```python
from build123d import *

# Parameters (mm, degrees)
SKETCH_1_R          = 22.25
SKETCH_1_R_2        = 2.5
EXTRUDE_1_DEPTH     = 2
SKETCH_3_R          = 11
SKETCH_3_R_2        = 2.5
EXTRUDE_3_DEPTH     = 13
EXTRUDE_START       = 6
SKETCH_4_R          = 11
EXTRUDE_4_DEPTH     = 6
SKETCH_6_R          = 2.5
CUT_EXTRUDE_2_DEPTH = 9


with BuildPart() as part:
    # 草图1 → 凸台-拉伸1 (new body)
    with BuildSketch(Plane(origin=(0, 0, 0), x_dir=(1, 0, 0), z_dir=(0, 1, 0))):
        with Locations(Location((0, 0, 0), (0, 0, 270))):
            Circle(SKETCH_1_R)
        with Locations(Location((0, 17.5, 0), (0, 0, 270))):
            Circle(SKETCH_1_R_2, mode=Mode.SUBTRACT)
        with Locations(Location((-15.155444566, -8.75, 0), (0, 0, 270))):
            Circle(SKETCH_1_R_2, mode=Mode.SUBTRACT)
        with Locations(Location((15.155444566, -8.75, 0), (0, 0, 270))):
            Circle(SKETCH_1_R_2, mode=Mode.SUBTRACT)
    extrude(amount=EXTRUDE_1_DEPTH)

    # 草图3 → 凸台-拉伸3 (add)
    with BuildSketch(Plane(origin=(0, 2, 0), x_dir=(1, 0, 0), z_dir=(0, 1, 0))):
        with Locations(Location((0, 0, 0), (0, 0, 90))):
            Circle(SKETCH_3_R)
        with Locations(Location((0, 0, 0), (0, 0, 90))):
            Circle(SKETCH_3_R_2, mode=Mode.SUBTRACT)
    extrude(amount=EXTRUDE_3_DEPTH)

    # 草图4 → 凸台-拉伸4 (add)
    with BuildSketch(Plane.XZ.offset(EXTRUDE_START)):
        with Locations(Location((0, 0, 0), (0, 0, 270))):
            Circle(SKETCH_4_R)
    extrude(amount=-EXTRUDE_4_DEPTH)

    # 草图6 → 切除-拉伸2 (cut)
    with BuildSketch(Plane.XZ.offset(6)):
        with Locations(Location((0, 0, 0), (0, 0, 270))):
            Circle(SKETCH_6_R)
    extrude(amount=-CUT_EXTRUDE_2_DEPTH, mode=Mode.SUBTRACT)


solid = part.part
```
Geometry: final body of the model. Coordinates: model frame, mm. A direction names the side the tool comes from. Give positions to 0.01 mm unless a question says otherwise; leave off trailing zeros. Loops run counter-clockwise (first coordinate to the right, second up) from the corner with the lowest first, then second, coordinate; pieces in that order, holes last. Notation, with made-up numbers: (-37.5, 17.25) -> (-6.5, 17.25) arc R24 cw to (-6.5, 49.25) -> close; hole circle Ø11 at (71.5, 75.25). An arc over 180 degrees is marked (long way). Return JSON: item names as keys, results as strings.
Item 1: Section D-D, the plane z = 8.75. Output: boundary loops of the cut face in (x, y), plus the area to 3 significant figures.
Filled in:
{"outline": "(-20.46, 0) -> (-17.66, 0) -> (-17.66, 2) -> (-20.46, 2) -> close; (-12.66, 0) -> (-6.67, 0) -> (-6.67, -6) -> (6.67, -6) -> (6.67, 0) -> (12.66, 0) -> (12.66, 2) -> (6.67, 2) -> (6.67, 15) -> (-6.67, 15) -> (-6.67, 2) -> (-12.66, 2) -> close; (17.66, 0) -> (20.46, 0) -> (20.46, 2) -> (17.66, 2) -> close", "area": "315 mm^2"}
Item 2: Pin query (flat end, axial travel): P1, Ø6, axis at x = 0, z = -17.5, coming from the +Y side; P2, Ø3, axis at x = 13.5, y = 7.5, coming from the +Z side; P3, Ø12, axis at y = 3, z = -15.5, coming from the +X side; P4, Ø1.5, axis at x = 9.5, y = 2, coming from the +Z side. Return the tip coordinate at first contact, or that it passes through.
Filled in:
{"P1": "y = 2", "P2": "through", "P3": "x = 20.08", "P4": "z = 20.46"}
Item 3: Section A-A, the plane z = 0. Output: boundary loops of the cut face in (x, y).
Filled in:
{"outline": "(-22.25, 0) -> (-11, 0) -> (-11, -6) -> (-2.5, -6) -> (-2.5, 15) -> (-11, 15) -> (-11, 2) -> (-22.25, 2) -> close; (2.5, -6) -> (11, -6) -> (11, 0) -> (22.25, 0) -> (22.25, 2) -> (11, 2) -> (11, 15) -> (2.5, 15) -> close"}
Item 4: Line query: line 1 (X direction, y = 8.25, z = 0); line 2 (X direction, y = 1.2, z = 8.75); line 3 (Y direction, x = 8, z = 8.5). Output: solid intervals per line, ascending.
Filled in:
{"line 1": "-11 to -2.5, 2.5 to 11", "line 2": "-20.46 to -17.66, -12.66 to 12.66, 17.66 to 20.46", "line 3": "0 to 2"}
Item 5: Mould query, pull axis X, two halves, no side actions, for faces 4 (the cylindrical face through (17.263, 0.986, 10.094)), 5 (the cylindrical face through (0, 1, -20)), 6 (the flat face through (-5, 2, -10)), 7 (the cylindrical face through (-10.74, -3.04, 2.38)). Classes: released by +X, released by -X, zero draft, split by the parting line, or undercut.
Filled in:
{"face 4": "undercut", "face 5": "undercut", "face 6": "zero draft", "face 7": "split by the parting line"}
Item 6: Access query for faces 1 (the cylindrical face through (10.74, 8.41, 2.38)), 2 (the flat face through (-5, 0, -10)), 3 (the flat face through (0, -6, 3)). Directions: +Z, -Z, +X, -X, +Y, -Y. A direction counts if a zero-diameter tool reaches every point of the face in a straight line with its end or side. Return the directions, or none.
Filled in:
{"face 1": "+Y", "face 2": "-Y", "face 3": "+Z, -Z, +X, -X, -Y"}
Item 7: Section B-B, the plane x = 0. Output: boundary loops of the cut face in (y, z), plus the area to 3 significant figures.
Filled in:
{"outline": "(-6, -11) -> (0, -11) -> (0, -15) -> (2, -15) -> (2, -11) -> (15, -11) -> (15, -2.5) -> (-6, -2.5) -> close; (-6, 2.5) -> (15, 2.5) -> (15, 11) -> (2, 11) -> (2, 22.25) -> (0, 22.25) -> (0, 11) -> (-6, 11) -> close; (0, -22.25) -> (2, -22.25) -> (2, -20) -> (0, -20) -> close", "area": "392 mm^2"}
Item 8: Section C-C, the plane y = 12.5. Output: boundary loops of the cut face in (x, z).
Filled in:
{"outline": "circle Ø22 at (0, 0); hole circle Ø5 at (0, 0)"}
